```python
from build123d import *

# Parameters (mm, degrees)
F1_DEPTH = 10
F2_DEPTH = 39
F3_R     = 1.27
F4_DEPTH = 39
F0_R     = 1.27
F5_DEPTH = 37


# Not quite as in the source:
# - a feature names something its author has since deleted; it is built from what else it names


with BuildPart() as f1:
    # F0 (on Top) → F1 (new body)
    with BuildSketch(Plane.XY):
        with BuildLine():
            Line((39.0916730868, 1.5), (-39.2084973779, 1.5))
            ThreePointArc((-39.2084973779, 1.5), (-39.0523737086, 0.7572105316), (-39, 0))
            ThreePointArc((-39, 0), (-39.0523737086, -0.7572105316), (-39.2084973779, -1.5))
            Line((-39.2084973779, -1.5), (35.8745669567, -1.5))
            Line((35.8745669567, -1.5), (39.0916730868, 1.5))
        make_face()
    extrude(amount=F1_DEPTH)

    # F0 (on Top) → F2 (join)
    with BuildSketch(Plane.XY):
        with BuildLine():
            ThreePointArc((-42.1130057398, -2.5597379557), (-47.0597379557, -2.3869942602), (-46.8869942602, 2.5597379557))
            Line((-46.8869942602, 2.5597379557), (-48.2509909803, 4.0224453589))
            ThreePointArc((-48.2509909803, 4.0224453589), (-48.5224453589, -3.7509909803), (-40.7490090197, -4.0224453589))
            Line((-40.7490090197, -4.0224453589), (-42.1130057398, -2.5597379557))
        make_face()
        with BuildLine():
            ThreePointArc((-46.8869942602, 2.5597379557), (-43.1043782588, 3.2097102603), (-41, 0))
            ThreePointArc((-41, 0), (-41.2902897397, -1.3956217412), (-42.1130057398, -2.5597379557))
            Line((-42.1130057398, -2.5597379557), (-40.7490090197, -4.0224453589))
            ThreePointArc((-40.7490090197, -4.0224453589), (-39.8061364224, -2.866643458), (-39.2084973779, -1.5))
            ThreePointArc((-39.2084973779, -1.5), (-39.0523737086, -0.7572105316), (-39, 0))
            ThreePointArc((-39, 0), (-39.0523737086, 0.7572105316), (-39.2084973779, 1.5))
            ThreePointArc((-39.2084973779, 1.5), (-43.0221716349, 5.2977375665), (-48.2509909803, 4.0224453589))
            Line((-48.2509909803, 4.0224453589), (-46.8869942602, 2.5597379557))
        make_face()
    extrude(amount=F2_DEPTH)

    # F3 (on face) → F4 (join)
    with BuildSketch(Plane.XY):
        with BuildLine():
            Line((-50.2566071407, -12.8884240397), (-40.7490090197, -4.0224453589))
            ThreePointArc((-40.7490090197, -4.0224453589), (-48.5224453589, -3.7509909803), (-48.2509909803, 4.0224453589))
            Line((-48.2509909803, 4.0224453589), (-57.7585891014, -4.8435333219))
            ThreePointArc((-57.7585891014, -4.8435333219), (-58.2346778018, -5.8882146293), (-57.8326221137, -6.9635614144))
            Line((-57.8326221137, -6.9635614144), (-52.3766352332, -12.8143910274))
            ThreePointArc((-52.3766352332, -12.8143910274), (-51.3319539259, -13.2904797278), (-50.2566071407, -12.8884240397))
        make_face()
        with Locations((-51.8135370162, -6.8199836006)):
            Circle(F3_R, mode=Mode.SUBTRACT)
    extrude(amount=F4_DEPTH)

    # F0 (on Top) → F5 (cut)
    with BuildSketch(Plane.XY):
        with BuildLine():
            ThreePointArc((-40.7490090197, -4.0224453589), (-48.5224453589, -3.7509909803), (-48.2509909803, 4.0224453589))
            Line((-48.2509909803, 4.0224453589), (-57.7585891014, -4.8435333219))
            ThreePointArc((-57.7585891014, -4.8435333219), (-58.2346778018, -5.8882146293), (-57.8326221137, -6.9635614144))
            Line((-57.8326221137, -6.9635614144), (-52.3766352332, -12.8143910274))
            ThreePointArc((-52.3766352332, -12.8143910274), (-51.3319539259, -13.2904797278), (-50.2566071407, -12.8884240397))
            Line((-50.2566071407, -12.8884240397), (-40.7490090197, -4.0224453589))
        make_face()
        with Locations((-51.8135370162, -6.8199836006)):
            Circle(F0_R, mode=Mode.SUBTRACT)
    extrude(amount=F5_DEPTH, mode=Mode.SUBTRACT)


solid = f1.part
```
Verification items for the finished model (mm, model axes). A direction names the side the tool comes from. Coordinates: 2 decimals unless noted, no trailing zeros. Write each loop counter-clockwise with the first axis right and the second up, starting at its lowest first coordinate (ties: lowest second). Pieces come first, ordered by that corner, then holes. Notation, with made-up numbers: M 66,9.5 L 80,9.5 A15 ccw 80,20.5 Z; hole C 13,82.5 d4. An arc over 180 degrees is marked long. One line per item, written item: value.
Item 1: Section check A-A, the plane z = 34. Record the boundary of the cut face in (x, y).
Check sheet entries:
outline: C -44.5,0 d11; hole C -44.5,0 d7
Item 2: Access from +Z, -Z, +X, -X, +Y, -Y to the whole of each face (thin tool, end or side, straight path). Record for faces 1 (the flat face through (-1, 0, 10)), 2 (the cylindrical face through (-51.35, -13.29, 37.99)), 3 (the flat face through (-12, 0, 0)), 4 (the flat face through (0, 1.5, 5)), 5 (the flat face through (-2, -1.5, 5)).
Check sheet entries:
face 1: +Z, +X, +Y, -Y
face 2: +Z, -Z, -Y
face 3: -Z, +X, -X, +Y, -Y
face 4: +Z, -Z, +X, +Y
face 5: +Z, -Z, +X, -Y
Item 3: Section check B-B, the plane x = -44.5. Record the boundary of the cut face in (y, z).
Check sheet entries:
outline: M -7.52,37 L -5.5,37 L -5.5,0 L -3.5,0 L -3.5,39 L -7.52,39 Z; M 3.5,0 L 5.5,0 L 5.5,39 L 3.5,39 Z
Item 4: Section check C-C, the plane z = 5. Record the boundary of the cut face in (x, y).
Check sheet entries:
outline: M -39.21,-1.5 L 35.87,-1.5 L 39.09,1.5 L -39.21,1.5 A5.5 ccw long Z; hole C -44.5,0 d7
Item 5: Mould release check, pull along Y, two halves, no side actions. Record for faces 6 (the cylindrical face through (-58.234, -5.872, 37.986)), 7 (the cylindrical face through (-53.082, -6.764, 37.986)), 8 (the flat face through (-55, -10, 38)), 9 (the flat face through (-49, -4, 39)): pulls with the +Y half, pulls with the -Y half, needs draft (parallel to the pull), parting line crosses it, or undercut.
Check sheet entries:
face 6: parting line crosses it
face 7: undercut
face 8: pulls with the -Y half
face 9: needs draft
Item 6: Section check D-D, the plane y = -10.5. Record the boundary of the cut face in (x, z).
Check sheet entries:
outline: M -54.53,37 L -47.7,37 L -47.7,39 L -54.53,39 Z
Item 7: Scan lines: line 1 along X through (y, z) = (0.25, 22.5); line 2 along Y through (x, z) = (11, 6); line 3 along X through (y, z) = (-3, 34). Record each from-to range of solid material in increasing order.
Check sheet entries:
line 1: x = -49.99 to -47.99, -41.01 to -39.01
line 2: y = -1.5 to 1.5
line 3: x = -49.11 to -46.3, -42.7 to -39.89
Item 8: Gauge pin test, flat ends, axial feed: pin 1 Ø2 at (x, y) = (12.5, -1) entering from -Z; pin 2 Ø0.9 at (x, y) = (7, 0) entering from +Z; pin 3 Ø2 at (y, z) = (-1.5, 31) entering from +X; pin 4 Ø3 at (x, z) = (16, 5) entering from +Y. Record the tip position at first contact, or that the pin passes through.
Check sheet entries:
pin 1: stops at z = 0
pin 2: stops at z = 10
pin 3: stops at x = -39.02
pin 4: stops at y = 1.5
